Input: part model. Units: mm. Frame: model coordinates. A direction names the side the tool comes from. Give positions to 0.01 mm unless a question says otherwise; leave off trailing zeros. Loops run counter-clockwise (first coordinate to the right, second up) from the corner with the lowest first, then second, coordinate; pieces in that order, holes last. Notation, with made-up numbers: (68, 24) - (89, 24) arc R5 cw to (89, 33) - close; hole circle Ø10 at (7.5, 7.25). An arc over 180 degrees is marked (long way). Answer as a JSON object with one key per item and string values.
from build123d import *

# Parameters (mm, degrees)
F1_DEPTH = 3.5
F3_DEPTH = 20
F5_DEPTH = 20


with BuildPart() as f1:
    # F0 (on Top) → F1 (new body)
    with BuildSketch(Plane.XY):
        with BuildLine():
            ThreePointArc((12.5, 20), (0, 32.5), (-12.5, 20))
            Line((-12.5, 20), (-12.5, -15))
            ThreePointArc((-12.5, -15), (0, -27.5), (12.5, -15))
            Line((12.5, -15), (12.5, 20))
        make_face()
    extrude(amount=F1_DEPTH)

    # F2 (on face) → F3 (join)
    with BuildSketch(Plane.XY.offset(3.5)):
        with BuildLine():
            ThreePointArc((9.871602, 18.500452), (-0.126027, 28.50059), (-10.128673, 18.50547))
            Line((-10.128673, 18.50547), (-10.128673, -13.49453))
            ThreePointArc((-10.128673, -13.49453), (-0.131046, -23.499687), (9.871602, -13.499548))
            Line((9.871602, -13.499548), (9.871602, 18.500452))
        make_face()
    extrude(amount=F3_DEPTH)

    # F4 (on face) → F5 (cut)
    with BuildSketch(Plane.XY.offset(23.5)):
        with BuildLine():
            ThreePointArc((-3.608536, 23.240072), (-5.374335, 21.156765), (-6.008536, 18.500452))
            Line((-6.008536, 18.500452), (-6.008536, -13.499548))
            ThreePointArc((-6.008536, -13.499548), (-4.553379, -17.371908), (-0.908138, -19.327637))
            Line((-0.908138, -19.327637), (-0.908138, -23.469252))
            ThreePointArc((-0.908138, -23.469252), (-0.035787, -24.319454), (0.821862, -23.454422))
            Line((0.821862, -23.454422), (0.821862, -19.302233))
            ThreePointArc((0.821862, -19.302233), (4.352688, -17.30652), (5.751464, -13.499548))
            Line((5.751464, -13.499548), (5.751464, 18.500452))
            ThreePointArc((5.751464, 18.500452), (5.117262, 21.156765), (3.351464, 23.240072))
            Line((3.351464, 23.240072), (3.351464, 27.875545))
            ThreePointArc((3.351464, 27.875545), (2.584662, 28.471802), (1.621464, 28.346277))
            Line((1.621464, 28.346277), (1.621464, 21.346277))
            Line((1.621464, 21.346277), (-1.878536, 21.346277))
            Line((-1.878536, 21.346277), (-1.878536, 28.346277))
            ThreePointArc((-1.878536, 28.346277), (-2.816511, 28.379103), (-3.608536, 27.875545))
            Line((-3.608536, 27.875545), (-3.608536, 23.240072))
        make_face()
    extrude(amount=-F5_DEPTH, mode=Mode.SUBTRACT)


solid = f1.part
Item 1: Cut plane C-C (x = -8). Return loops of the section in (y, z), then the cut area to 3 significant figures.
Geometry check:
{"outline": "(-24.6, 0) - (29.6, 0) - (29.6, 3.5) - (24.67, 3.5) - (24.67, 23.5) - (-19.67, 23.5) - (-19.67, 3.5) - (-24.6, 3.5) - close", "area": "1,080 mm2"}
Item 2: Contact query for flat-ended pins moving along their axis: P1, Ø1.5, axis at x = -1, y = 19.5, coming from the -Z side; P2, Ø3, axis at y = -11, z = 17.5, coming from the +X side; P3, Ø2, axis at x = 3.5, z = 7.5, coming from the -Y side; P4, Ø7.5, axis at y = 25.5, z = 12.5, coming from the -X side. Output: stop coordinate, or through.
Geometry check:
{"P1": "stops at z = 0", "P2": "stops at x = 9.87", "P3": "stops at y = -23.15", "P4": "stops at x = -9.59"}
Item 3: Cut plane D-D (z = 2.25). Return loops of the section in (x, y).
Geometry check:
{"outline": "(-12.5, -15) arc R12.5 ccw to (12.5, -15) - (12.5, 20) arc R12.5 ccw to (-12.5, 20) - close"}
Item 4: Access query for faces 4 (the face through (-10.129, 3, 13)), 5 (the face through (0.822, -21, 14)), 6 (the face through (-4.59, -17.33, 13.64)), 7 (the face through (8.13, 24.14, 13.36)), 8 (the face through (-3.609, 26, 14)). Directions: +Z, -Z, +X, -X, +Y, -Y. A direction counts if a zero-diameter tool reaches every point of the face in a straight line with its end or side. Return the directions, or none.
Geometry check:
{"face 4": "+Z, -X, +Y, -Y", "face 5": "+Z, -Y", "face 6": "+Z", "face 7": "+Z, +X, +Y", "face 8": "+Z, +Y"}
Item 5: Material intervals for line 1 (X direction, y = -5.5, z = 14); line 2 (X direction, y = 27.5, z = 4.75); line 3 (X direction, y = 27, z = 20), sorted ascending. Write a range as [from, to].
Geometry check:
{"line 1": "x = [-10.13, -6.01], [5.75, 9.87]", "line 2": "x = [-4.49, -3.61], [-1.88, 1.62], [3.35, 4.23]", "line 3": "x = [-5.4, -3.61], [-1.88, 1.62], [3.35, 5.14]"}
Item 6: Cut plane B-B (y = 3). Return loops of the section in (x, z).
Geometry check:
{"outline": "(-12.5, 0) - (12.5, 0) - (12.5, 3.5) - (9.87, 3.5) - (9.87, 23.5) - (5.75, 23.5) - (5.75, 3.5) - (-6.01, 3.5) - (-6.01, 23.5) - (-10.13, 23.5) - (-10.13, 3.5) - (-12.5, 3.5) - close"}
Item 7: Mould query, pull axis Y, two halves, no side actions, for faces 1 (the face through (0, 21.346, 14)), 2 (the face through (0.275, 32.497, 1.726)), 3 (the face through (9.872, 2, 13)). Classes: released by +Y, released by -Y, zero draft, split by the parting line, or undercut.
Geometry check:
{"face 1": "undercut", "face 2": "released by +Y", "face 3": "zero draft"}
